Geometry check sheet. Reference: the model listing, model coordinates, mm. Face numbers are marked on the shaded views. A direction names the side the tool comes from. Round coordinates to 2 decimals unless told otherwise and drop trailing zeros. Write each loop counter-clockwise with the first axis right and the second up, starting at its lowest first coordinate (ties: lowest second). Pieces come first, ordered by that corner, then holes. Notation, with made-up numbers: (-18, -18.75) - (-14, -18.75) arc R35 cw to (-14, 16.25) - close; hole circle Ø11 at (68, 54.25). An arc over 180 degrees is marked (long way). Return JSON: item names as keys, results as strings.
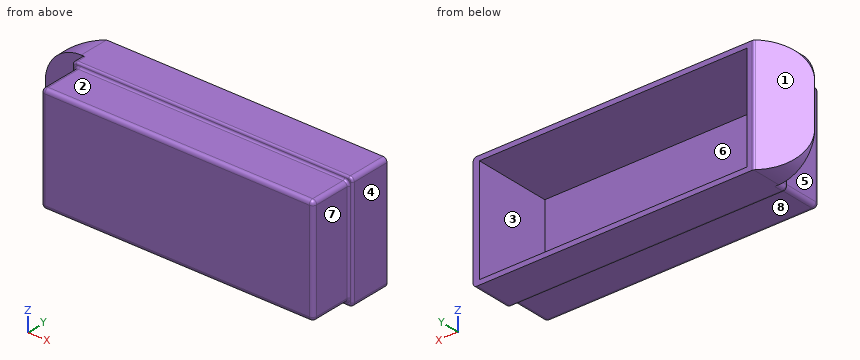
```python
from build123d import *

# Parameters (mm, degrees)
SKETCH1_W           = 139.7
SKETCH1_H           = 57.15
BOSS_EXTRUDE1_DEPTH = 20.32
SKETCH2_W           = 135.7
SKETCH2_H           = 53.15
BOSS_EXTRUDE2_DEPTH = 20.955
BOSS_EXTRUDE3_DEPTH = 57.15
CUT_EXTRUDE1_DEPTH  = 96.931280842
FILLET1_R           = 2
FILLET2_R           = 1
SKETCH5_W           = 133.35
SKETCH5_H           = 52.35
CUT_EXTRUDE2_DEPTH  = 38.735


with BuildPart() as part:
    # Sketch1 → Boss-Extrude1 (new body)
    with BuildSketch(Plane(origin=(0, 0, 0), x_dir=(1, 0, 0), z_dir=(0, 1, 0))):
        Rectangle(SKETCH1_W, SKETCH1_H)
    extrude(amount=BOSS_EXTRUDE1_DEPTH)

    # Sketch2 → Boss-Extrude2 (add)
    with BuildSketch(Plane.XZ):
        Rectangle(SKETCH2_W, SKETCH2_H)
    extrude(amount=BOSS_EXTRUDE2_DEPTH)

    # Sketch3 → Boss-Extrude3 (add, through all)
    with BuildSketch(Plane.XY.offset(28.575)):
        Polygon((-69.85, 20.32), (-87.726303889, 5.32), (-69.85, 5.32), align=None)
    extrude(amount=-BOSS_EXTRUDE3_DEPTH)

    # Sketch4 → Cut-Extrude1 (cut, through all)
    with BuildSketch(Plane.XZ.offset(-5.32)):
        with BuildLine():
            Line((-69.85, -28.575), (-87.726303889, -28.575))
            Line((-87.726303889, -28.575), (-87.726303889, -10.698696111))
            ThreePointArc((-87.726303889, -10.698696111), (-82.490455702, -23.339151813), (-69.85, -28.575))
        make_face()
        with BuildLine():
            Line((-87.726303889, 10.698696111), (-87.726303889, 28.575))
            Line((-87.726303889, 28.575), (-69.85, 28.575))
            ThreePointArc((-69.85, 28.575), (-82.490455702, 23.339151813), (-87.726303889, 10.698696111))
        make_face()
    extrude(amount=-CUT_EXTRUDE1_DEPTH, mode=Mode.SUBTRACT)

    # Fillet1
    fillet1_edges = [part.edges().sort_by_distance(p)[0] for p in [
        (-69.85, 20.32, 0),
        (-69.85, 2.66, -28.575),
        (-67.85, -10.4775, -26.575),
        (69.85, 10.16, -28.575),
        (67.85, -10.4775, -26.575),
        (69.85, 10.16, 28.575),
        (67.85, -10.4775, 26.575),
        (-67.85, -10.4775, 26.575),
        (-69.85, 2.66, 28.575),
        (-67.85, -20.955, 0),
        (0, -20.955, 26.575),
        (67.85, -20.955, 0),
        (0, -20.955, -26.575),
    ]]
    fillet(fillet1_edges, radius=FILLET1_R)

    # Fillet2
    fillet2_edges = [part.edges().sort_by_distance(p)[0] for p in [
        (0, 0, 28.575),
        (0, 0, -28.575),
        (-67.85, 0, 0),
        (0, 0, 26.575),
        (67.85, 0, 0),
        (0, 0, -26.575),
        (-69.85, 0, 0),
        (69.85, 0, 0),
        (-69.264213562, 0, 27.989213562),
        (69.264213562, 0, 27.989213562),
        (69.264213562, 0, -27.989213562),
        (-69.264213562, 0, -27.989213562),
        (-67.264213562, 0, -25.989213562),
        (67.264213562, 0, -25.989213562),
        (67.264213562, 0, 25.989213562),
        (-67.264213562, 0, 25.989213562),
    ]]
    fillet(fillet2_edges, radius=FILLET2_R - 0.0001)  # a hair under: the kernel refuses the full size

    # Sketch5 → Cut-Extrude2 (cut)
    with BuildSketch(Plane(origin=(0, 20.32, 0), x_dir=(1, 0, 0), z_dir=(0, 1, 0))):
        Rectangle(SKETCH5_W, SKETCH5_H)
    extrude(amount=-CUT_EXTRUDE2_DEPTH, mode=Mode.SUBTRACT)


solid = part.part
```
(1) Gauge pin test, flat ends, axial feed: pin 1 (20 mm diameter, centred on x = 8, y = -11.5, fed in from -Z) (3 decimals); pin 2 (5 mm diameter, centred on y = -8.5, z = 14, fed in from +X); pin 3 (9 mm diameter, centred on x = 11, y = -14, fed in from +Z) (3 decimals). Record the tip position at first contact, or that the pin passes through.
Response values:
{"pin 1": "stops at z = -26.575", "pin 2": "stops at x = 67.85", "pin 3": "stops at z = 26.575"}
(2) Release check for a two-part mould opening along Z. For the marked faces 1, 2 and 3 record: pulls with the +Z half, pulls with the -Z half, needs draft (parallel to the pull), parting line crosses it, or undercut.
Response values:
{"face 1": "needs draft", "face 2": "pulls with the +Z half", "face 3": "undercut"}
(3) Access from +Z, -Z, +X, -X, +Y, -Y to the whole of each face (thin tool, end or side, straight path). Record for the marked faces 4, 5, 6, 7 and 8.
Response values:
{"face 4": "+Z, -Z, +X, +Y, -Y", "face 5": "+Z, -Z, -X, -Y", "face 6": "+Y", "face 7": "+Z, -Z, +X, -Y", "face 8": "-Z, +X, -X, -Y"}
(4) Material ranges on line 1 along Z through (x, y) = (-34, -9) (3 decimals); line 2 along Z through (x, y) = (10.5, 5.5) (3 decimals); line 3 along X through (y, z) = (-6, 2) (3 decimals), recorded low to high. Write a range as [from, to].
Response values:
{"line 1": "z = [-26.575, -26.175], [26.175, 26.575]", "line 2": "z = [-28.575, -26.175], [26.175, 28.575]", "line 3": "x = [-67.85, -66.675], [66.675, 67.85]"}
(5) Section check A-A, the plane y = -6. Enter the section's corners in (x, z) (3 decimals).
Response values:
{"outline": "(-67.85, -24.575) arc R2 ccw to (-65.85, -26.575) - (65.85, -26.575) arc R2 ccw to (67.85, -24.575) - (67.85, 24.575) arc R2 ccw to (65.85, 26.575) - (-65.85, 26.575) arc R2 ccw to (-67.85, 24.575) - close; hole (-66.675, -26.175) - (66.675, -26.175) - (66.675, 26.175) - (-66.675, 26.175) - close"}
